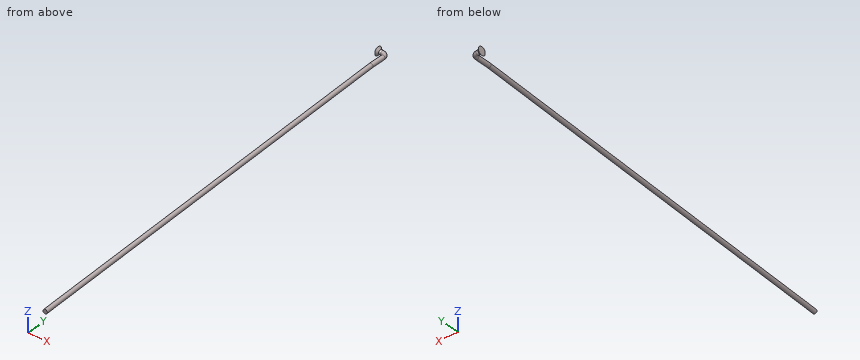
from build123d import *

# Parameters (mm, degrees)
ESQUISSE2_R = 1


with BuildPart() as part:
    # Balayage1: sweep along a path in Esquisse1
    with BuildLine(Plane.XY) as balayage1_path:
        Line((-4, 0), (-2, 0))
        ThreePointArc((-2, 0), (-0.585786438, -0.585786438), (0, -2))
        Line((0, -2), (0, -9))
        Line((0, -9), (10.52014508, -209.736326247))
    # Esquisse2 → Balayage1 (sweep)
    with BuildSketch(Plane(origin=(-4, 0, 0), x_dir=(0, 0, -1), z_dir=(1, 0, 0))):
        Circle(ESQUISSE2_R)
    sweep(path=balayage1_path.line, transition=Transition.RIGHT)

    # Esquisse3 → Révolution1 (revolve)
    with BuildSketch(Plane.XY):
        Polygon((-4, 1), (-4, 2), (-3, 1), align=None)
    revolve(axis=Axis((0, 0, 0), (-1, 0, 0)))


solid = part.part
The model under review builds one solid part; all positions refer to its coordinate system, in mm. Round coordinates to 2 decimals unless told otherwise and drop trailing zeros. Loops run counter-clockwise (first coordinate to the right, second up) from the corner with the lowest first, then second, coordinate; pieces in that order, holes last. Notation, with made-up numbers: (9, -19) -> (54, -19) arc R21 ccw to (54, -1) -> close; hole circle Ø7 at (-20.75, 78.5). An arc over 180 degrees is marked (long way). Return JSON: item names as keys, results as strings.
(1) For line 1 (X direction, y = -85.5, z = -0.75); line 2 (X direction, y = -78, z = -0.3); line 3 (Z direction, x = 6, y = -139), list the stretches that pass through material, from the lowest coordinate up.
Solved:
{"line 1": "3.35 to 4.67", "line 2": "2.66 to 4.57", "line 3": "-0.58 to 0.58"}
(2) For pin 1 (2 mm diameter, centred on y = -94.5, z = -0.5, fed in from -X); pin 2 (1 mm diameter, centred on y = -174.5, z = 0, fed in from -X), all flat-tipped, find the tip position at first contact; note any pin that passes through.
Solved:
{"pin 1": "x = 3.43", "pin 2": "x = 7.65"}
(3) Add section A-A on z = 0. Write out the cut boundary in (x, y), plus the area to 3 significant figures.
Solved:
{"outline": "(-4, -2) -> (-3, -1) -> (-2, -1) arc R1 cw to (-1, -2) -> (-1, -9.03) -> (9.52, -209.79) -> (11.52, -209.68) -> (1, -8.97) -> (1, -2) arc R3 ccw to (-2, 1) -> (-3, 1) -> (-4, 2) -> close", "area": "427 mm2"}
